The listing builds one solid part. Answer for the finished solid, in the listing's coordinates (mm). A direction names the side the tool comes from. Coordinates: 2 decimals unless noted, no trailing zeros. Order: outer loops, then holes, each group sorted by start corner. A loop starts at its lowest first (then second) coordinate and runs counter-clockwise, first axis right, second up. Notation, with made-up numbers: (-33.75, -20.5) -> (-29.75, -20.5) arc R13 cw to (-29.75, -11.5) -> close; hole circle Ø7 at (-31.75, 3). An arc over 180 degrees is marked (long way). Answer in a Markdown table with one row per item.
```python
from build123d import *

# Parameters (mm, degrees)
F1_DEPTH = 31.75
F2_R     = 12.7
F3_DEPTH = 1320.8
F4_R     = 12.7
F5_DEPTH = 101.6


with BuildPart() as f1:
    # F0 (on Right) → F1 (new body)
    with BuildSketch(Plane.YZ):
        Polygon((-25.733576, 56.262951), (-53.673576, 56.262951), (-53.673576, 0.382951), (-25.733576, 0.382951), (-25.733576, 28.322951), (2.206424, 28.322951), (2.206424, 56.262951), align=None)
    extrude(amount=F1_DEPTH)

    # F2 (on face) → F3 (join)
    with BuildSketch(Plane(origin=(0, 2.206424, 0), x_dir=(-1, 0, 0), z_dir=(0, 1, 0))):
        with Locations((-15.875, 42.292951)):
            Circle(F2_R)
    extrude(amount=F3_DEPTH)

    # F4 (on face) → F5 (join)
    with BuildSketch(Plane(origin=(0, 0, 0.382951), x_dir=(1, 0, 0), z_dir=(0, 0, -1))):
        with Locations((15.875, 39.703576)):
            Circle(F4_R)
    extrude(amount=F5_DEPTH)


solid = f1.part
```
(1) Flat-ended cylindrical pins translate along their axes: pin 1 (6 mm diameter, centred on x = 18, y = 810, fed in from +Z); pin 2 (10 mm diameter, centred on x = 23.5, y = 151.5, fed in from +Z); pin 3 (4 mm diameter, centred on x = 24.5, y = 921, fed in from -Z). Find the tip coordinate at first contact, or state that the pin passes through.
Check values:
| item | result |
|---|---|
| pin 1 | z = 54.99 |
| pin 2 | z = 54.72 |
| pin 3 | z = 31.46 |
(2) Which of the six approach directions +Z, -Z, +X, -X, +Y, -Y give full straight-line access (tool end or side, diameter ignored) to faces 1 (the flat face through (12, -52, 0.383)), 2 (the flat face through (0, -32, 35)), 3 (the cylindrical face through (17.528, 653.361, 54.885)), 4 (the flat face through (16, -25.734, 14))?
Check values:
| item | result |
|---|---|
| face 1 | -Z |
| face 2 | +Z, -Z, -X, +Y, -Y |
| face 3 | +Y |
| face 4 | -Z, +X, -X, +Y |
(3) A cutting plane is placed at C-C, the plane z = -20.5. Determine the outline of the cut face in (x, y) (3 decimals).
Check values:
| item | result |
|---|---|
| outline | circle Ø25.4 at (15.875, -39.704) |
(4) A cutting plane is placed at B-B, the plane y = 521. Determine the outline of the cut face in (x, z) (3 decimals).
Check values:
| item | result |
|---|---|
| outline | circle Ø25.4 at (15.875, 42.293) |
(5) A cutting plane is placed at A-A, the plane x = 10.5. Determine the outline of the cut face in (y, z), then the cut area to 3 significant figures.
Check values:
| item | result |
|---|---|
| outline | (-53.67, 0.38) -> (-51.21, 0.38) -> (-51.21, -101.22) -> (-28.2, -101.22) -> (-28.2, 0.38) -> (-25.73, 0.38) -> (-25.73, 28.32) -> (2.21, 28.32) -> (2.21, 30.79) -> (1323.01, 30.79) -> (1323.01, 53.8) -> (2.21, 53.8) -> (2.21, 56.26) -> (-53.67, 56.26) -> close |
| area | 35,100 mm² |
(6) Find the intervals of material crossed by line 1 along Z through (x, y) = (14, 789.5); line 2 along X through (y, z) = (186, 44); line 3 along Y through (x, z) = (5.5, 22), in increasing order. Write a range as from..to.
Check values:
| item | result |
|---|---|
| line 1 | 29.73..54.85 |
| line 2 | 3.29..28.46 |
| line 3 | -53.67..-25.73 |
